CAD build for the part. Positions are in the model's coordinates, mm. Round coordinates to 2 decimals unless told otherwise and drop trailing zeros. Loops run counter-clockwise (first coordinate to the right, second up) from the corner with the lowest first, then second, coordinate; pieces in that order, holes last. Notation, with made-up numbers: (-33, -18.5) - (-10, -18.5) arc R25 ccw to (-10, -4.5) - close; hole circle Ø11 at (4, 52). An arc over 180 degrees is marked (long way). Use one line per item in the form item = value.
from build123d import *

# Parameters (mm, degrees)
CROQUIS2_W              = 1
CROQUIS2_H              = 400
SALIENTE_EXTRUIR2_DEPTH = 25
CROQUIS5_R              = 1.5
CORTAR_EXTRUIR2_DEPTH   = 1
CROQUIS1_R              = 1.5
SALIENTE_EXTRUIR3_DEPTH = 1


with BuildPart() as part:
    # Croquis2 → Saliente-Extruir2 (new body)
    with BuildSketch(Plane.XY):
        with Locations((-54.941785307, -92.819624774)):
            Rectangle(CROQUIS2_W, CROQUIS2_H)
    extrude(amount=SALIENTE_EXTRUIR2_DEPTH)

    # Croquis5 → Cortar-Extruir2 (cut)
    with BuildSketch(Plane(origin=(-54.441785307, 0, 0), x_dir=(0, 0, -1), z_dir=(1, 0, 0))):
        with Locations((-20, 89.180375226)):
            Circle(CROQUIS5_R)
        with Locations((-20, -274.819624774)):
            Circle(CROQUIS5_R)
        with Locations((-20, -92.819624774)):
            Circle(CROQUIS5_R)
    extrude(amount=-CORTAR_EXTRUIR2_DEPTH, mode=Mode.SUBTRACT)

    # Croquis1 → Saliente-Extruir3 (add)
    with BuildSketch(Plane.XY):
        Polygon((-79.441785307, 83.180375226), (-79.441785307, -268.819624774), (-55.441785307, -292.819624774), (-55.441785307, 107.180375226), align=None)
        with Locations((-74.441785307, 47.180375226)):
            Circle(CROQUIS1_R, mode=Mode.SUBTRACT)
        with Locations((-74.441785307, -232.819624774)):
            Circle(CROQUIS1_R, mode=Mode.SUBTRACT)
    extrude(amount=SALIENTE_EXTRUIR3_DEPTH)


solid = part.part
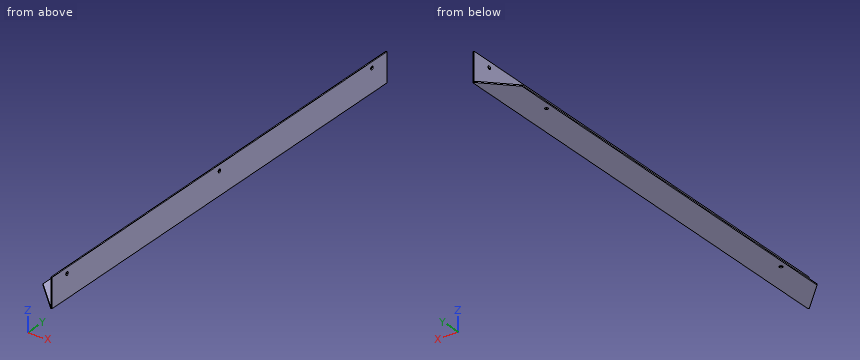
1) Slice it at A-A (y = 54). Write the cut outline in (x, z), plus the area to 3 significant figures.
Report:
outline = (-79.44, 0) - (-54.44, 0) - (-54.44, 25) - (-55.44, 25) - (-55.44, 1) - (-79.44, 1) - close
area = 49.0 mm^2
2) Drill centre lines: probe 1 along X at (y, z) = (-237, 20); probe 2 along Z at (x, y) = (-70.5, -54). Where is each one in solid material? Low to high.
Report:
probe_1 = -55.44 to -54.44
probe_2 = 0 to 1
3) Slice it at C-C (x = -65.5). Write the cut outline in (y, z).
Report:
outline = (-282.76, 0) - (97.12, 0) - (97.12, 1) - (-282.76, 1) - close
4) Flat gauge pins, fed straight in: pin 1 (2 mm diameter, centred on x = -74.5, y = -233.5, fed in from +Z); pin 2 (3.5 mm diameter, centred on y = -274.82, z = 20, fed in from +X); pin 3 (1 mm diameter, centred on y = 23, z = 3, fed in from -X). Where does each tip first touch, or does it go through?
Report:
pin_1 = 1
pin_2 = -54.44
pin_3 = -55.44
5) Slice it at B-B (z = 6.75). Write the cut outline in (x, y).
Report:
outline = (-55.44, -292.82) - (-54.44, -292.82) - (-54.44, 107.18) - (-55.44, 107.18) - close
